Can you work these out from the model? Positions are in its coordinate system, mm. Face numbers are marked on the shaded views. A direction names the side the tool comes from. Round coordinates to 2 decimals unless told otherwise and drop trailing zeros. Loops run counter-clockwise (first coordinate to the right, second up) from the corner with the lowest first, then second, coordinate; pieces in that order, holes last. Notation, with made-up numbers: M 55.5,50.5 L 77.5,50.5 A21 ccw 77.5,76.5 Z; hole C -37,-19 d10. An arc over 180 degrees is marked long. Return JSON: item names as keys, results as strings.
```python
from build123d import *

# Parameters (mm, degrees)
SKETCH1_W               = 50
SKETCH1_H               = 50
BOSS_EXTRUDE1_DEPTH     = 650
SKETCH2_W               = 450
SKETCH2_H               = 600
BOSS_EXTRUDE2_DEPTH     = 25
SKETCH4_W               = 450
SKETCH4_H               = 30
BOSS_EXTRUDE3_DEPTH     = 60
SKETCH5_R               = 10
CUT_EXTRUDE1_DEPTH      = 510
SKETCH7_W               = 50
SKETCH7_H               = 20
BOSS_EXTRUDE4_DEPTH     = 58
SKETCH8_R               = 10
CUT_EXTRUDE3_DEPTH      = 635
CUT_EXTRUDE3_DEPTH_BACK = 20
SKETCH9_W               = 30
SKETCH9_H               = 90
BOSS_EXTRUDE5_DEPTH     = 60
SKETCH10_R              = 10
CUT_EXTRUDE4_DEPTH      = 214


with BuildPart() as part:
    # Sketch1 → Boss-Extrude1 (new body)
    with BuildSketch(Plane.XY):
        with Locations((-10.215053763, 2.150537634)):
            Rectangle(SKETCH1_W, SKETCH1_H)
    extrude(amount=BOSS_EXTRUDE1_DEPTH)

    # Sketch2 → Boss-Extrude2 (add)
    with BuildSketch(Plane.XY.offset(650)):
        with Locations((-10.215053763, -262.849462366)):
            Rectangle(SKETCH2_W, SKETCH2_H)
    extrude(amount=BOSS_EXTRUDE2_DEPTH)

    # Sketch4 → Boss-Extrude3 (add)
    with BuildSketch(Plane(origin=(0, 0, 650), x_dir=(-1, 0, 0), z_dir=(0, 0, -1))):
        with Locations((10.215053763, -547.849462366)):
            Rectangle(SKETCH4_W, SKETCH4_H)
        with Locations((10.215053763, -67.849462366)):
            Rectangle(SKETCH4_W, SKETCH4_H)
    extrude(amount=BOSS_EXTRUDE3_DEPTH)

    # Sketch5 → Cut-Extrude1 (cut)
    with BuildSketch(Plane.XZ.offset(562.849462366)):
        with Locations((-10.215053763, 625)):
            Circle(SKETCH5_R)
    extrude(amount=-CUT_EXTRUDE1_DEPTH, mode=Mode.SUBTRACT)

    # Sketch7 → Boss-Extrude4 (add)
    with BuildSketch(Plane.XZ.offset(22.849462366)):
        with Locations((-10.215053763, 10)):
            Rectangle(SKETCH7_W, SKETCH7_H)
    extrude(amount=BOSS_EXTRUDE4_DEPTH)

    # Sketch8 → Cut-Extrude3 (cut, two sides)
    with BuildSketch(Plane(origin=(0, 0, 650), x_dir=(-1, 0, 0), z_dir=(0, 0, -1))) as cut_extrude3_sk:
        with Locations((10.215053763, -41.849462366)):
            Circle(SKETCH8_R)
    extrude(amount=CUT_EXTRUDE3_DEPTH, mode=Mode.SUBTRACT)
    extrude(cut_extrude3_sk.sketch, amount=-CUT_EXTRUDE3_DEPTH_BACK, mode=Mode.SUBTRACT)

    # Sketch9 → Boss-Extrude5 (add)
    with BuildSketch(Plane(origin=(0, 0, 650), x_dir=(-1, 0, 0), z_dir=(0, 0, -1))):
        with Locations((-199.784946237, -7.849462366)):
            Rectangle(SKETCH9_W, SKETCH9_H)
    extrude(amount=BOSS_EXTRUDE5_DEPTH)

    # Sketch10 → Cut-Extrude4 (cut)
    with BuildSketch(Plane(origin=(214.784946237, 0, 0), x_dir=(0, 0, -1), z_dir=(1, 0, 0))):
        with Locations((-625, 0)):
            Circle(SKETCH10_R)
    extrude(amount=-CUT_EXTRUDE4_DEPTH, mode=Mode.SUBTRACT)


solid = part.part
```
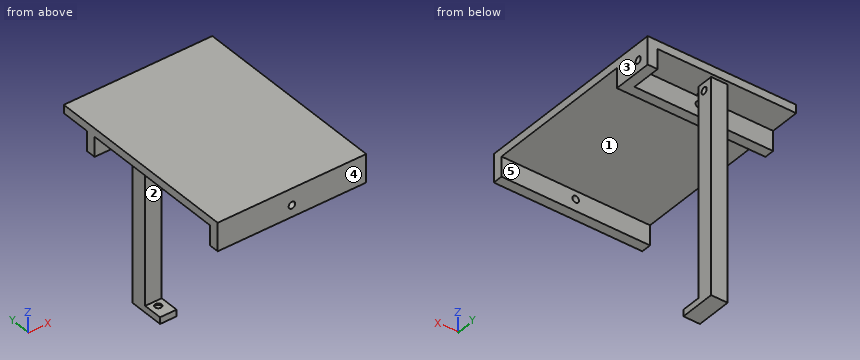
Q1. Suppose I cut it at C-C, the plane x = 54. Please give me the cut outline in (y, z), plus the area to 3 significant figures.
Results:
{"outline": "M -562.85,590 L -532.85,590 L -532.85,650 L -82.85,650 L -82.85,590 L -52.85,590 L -52.85,650 L 37.15,650 L 37.15,675 L -562.85,675 Z", "area": "18,600 mm2"}
Q2. Suppose I cut it at B-B, the plane z = 625. State how many separate pieces and enclosed holes the cut face has, plus the area to 3 significant figures.
Results:
{"separate pieces": "6", "enclosed holes": "0", "area": "30,100 mm2"}
Q3. I'm going to push flat-ended pins straight in: pin 1 Ø12 at (x, z) = (-10.22, 625) entering from -Y; pin 2 Ø1 at (x, y) = (110.5, -74.5) entering from -Z; pin 3 Ø23 at (y, z) = (0, 625) entering from -X. Where does each tip first touch, or does it pass through?
Results:
{"pin 1": "stops at y = -22.85", "pin 2": "stops at z = 590", "pin 3": "stops at x = -35.22"}
Q4. On a 3-axis mill with a long thin cutter (end or side, diameter ignored), from which of +Z, -Z, +X, -X, +Y, -Y can I reach the whole of each face in a straight line? I mean the marked faces 4 and 5. Say none if no direction works.
Results:
{"face 4": "+Z, -Z, +X, -X, -Y", "face 5": "-Z, +X, -X"}
Q5. If I drill on line 1 along Y through (x, z) = (6, 625); line 2 along X through (y, z) = (-541, 625); line 3 along Z through (x, y) = (-135, -191.5), over which ranges is the centre line in solid material (lowest first)?
Results:
{"line 1": "y = -562.85 to -532.85, -82.85 to -52.85, -22.85 to -10, 10 to 27.15", "line 2": "x = -235.22 to -20.22, -0.22 to 214.78", "line 3": "z = 650 to 675"}
Q6. Suppose I cut it at D-D, the plane z = 194.5. Please give me the cut outline in (x, y).
Results:
{"outline": "M -35.22,-22.85 L 14.78,-22.85 L 14.78,27.15 L -35.22,27.15 Z"}
Q7. Thinking about a two-plate mould opening in Z: for the marked faces 1, 2 and 3, which applies, pulls with the +Z half, pulls with the -Z half, needs draft (parallel to the pull), parting line crosses it, or undercut?
Results:
{"face 1": "pulls with the -Z half", "face 2": "undercut", "face 3": "needs draft"}
Q8. Suppose I cut it at A-A, the plane y = 0. Please give me the cut outline in (x, z), plus the area to 3 significant figures.
Results:
{"outline": "M -235.22,650 L -35.22,650 L -35.22,0 L 14.78,0 L 14.78,615 L 0.78,615 L 0.78,635 L 14.78,635 L 14.78,650 L 184.78,650 L 184.78,635 L 214.78,635 L 214.78,675 L -235.22,675 Z; M 184.78,590 L 214.78,590 L 214.78,615 L 184.78,615 Z", "area": "44,700 mm2"}
